Input: part model. Units: mm. Frame: model coordinates. A direction names the side the tool comes from. Give positions to 0.01 mm unless a question says otherwise; leave off trailing zeros. Loops run counter-clockwise (first coordinate to the right, second up) from the corner with the lowest first, then second, coordinate; pieces in that order, holes last. Notation, with made-up numbers: (13, 71) -> (33, 71) arc R21 cw to (33, 89) -> close; hole circle Ø9 at (-11, 82). An arc over 180 degrees is marked (long way). Answer as a JSON object with one key per item and string values.
```python
from build123d import *

# Parameters (mm, degrees)
F3_DEPTH = 1.27


with BuildPart() as f1:
    # F0 (on Front) → F1 (revolve)
    with BuildSketch(Plane.XZ):
        with BuildLine():
            Line((1.389063, -9.525), (1.389063, 0))
            Line((1.389063, 0), (3.3274, 0))
            ThreePointArc((3.3274, 0), (2.573122, 1.099922), (1.4732, 1.8542))
            Line((1.4732, 1.8542), (0, 1.8542))
            Line((0, 1.8542), (0, 0))
            Line((0, 0), (0, -9.525))
            Line((0, -9.525), (1.389063, -9.525))
        make_face()
    revolve(axis=Axis((0, 0, -4.7625), (0, 0, -1)))

    # F2 (on face) → F3 (cut)
    with BuildSketch(Plane.XY.offset(1.8542)):
        Polygon((0.57284, 0.992188), (-0.57284, 0.992188), (-1.145679, 0), (-0.57284, -0.992188), (0.57284, -0.992188), (1.145679, 0), align=None)
    extrude(amount=-F3_DEPTH, mode=Mode.SUBTRACT)


solid = f1.part
```
Q1. Ray query, line 1 along X through (y, z) = (0, -7.25); line 2 along Z through (x, y) = (1.5, -0.5); line 3 along X through (y, z) = (-1.25, -2). Return the intervals inside material, ascending.
Evaluation:
{"line 1": "x = -1.39 to 1.39", "line 2": "z = 0 to 1.8", "line 3": "x = -0.61 to 0.61"}
Q2. Pin query (flat end, axial travel): pin 1 (0.6 mm diameter, centred on x = -0.5, z = 1, fed in from -Y); pin 2 (2 mm diameter, centred on y = 0, z = -3, fed in from -X); pin 3 (1.3 mm diameter, centred on x = 0, z = 1, fed in from +Y). Return the tip coordinate at first contact, or that it passes through.
Evaluation:
{"pin 1": "stops at y = -2.88", "pin 2": "stops at x = -1.39", "pin 3": "stops at y = 3.15"}
Q3. Access query for faces 5 (the flat face through (-0.855, 0.503, 1.228)), 6 (the flat face through (0, 0, -9.525)). Directions: +Z, -Z, +X, -X, +Y, -Y. A direction counts if a zero-diameter tool reaches every point of the face in a straight line with its end or side. Return the directions, or none.
Evaluation:
{"face 5": "+Z", "face 6": "-Z, +X, -X, +Y, -Y"}
Q4. Draft query along X for faces 1 (the flat face through (0.855, -0.503, 1.228)), 2 (the flat face through (-1.4, 0.7, 0)), 3 (the cylindrical face through (-0.301, 1.356, -4.696)), 4 (the flat face through (-0.863, -0.489, 1.228)). Return one class per face: +X half, -X half, draft (parallel to the pull), parting line (faces both ways), or undercut.
Evaluation:
{"face 1": "undercut", "face 2": "draft", "face 3": "parting line", "face 4": "undercut"}
Q5. Section A-A, the plane z = -4. Return the cut outline in (x, y), then the cut area to 3 significant figures.
Evaluation:
{"outline": "circle Ø2.78 at (0, 0)", "area": "6.06 mm2"}
